Source: CAD feature listing. Evaluate the final solid. Frame: model axes, mm. Face numbers are marked on the shaded views. Coordinates: 2 decimals unless noted, no trailing zeros. Order: outer loops, then holes, each group sorted by start corner. A loop starts at its lowest first (then second) coordinate and runs counter-clockwise, first axis right, second up. Notation, with made-up numbers: (-4, 27) -> (41, 27) arc R25 ccw to (41, 47) -> close; hole circle Ø1 at (-17, -3.75). An arc over 180 degrees is marked (long way). Put each result on its own line as item: value.
from build123d import *

# Parameters (mm, degrees)
F1_DEPTH       = 3.175
F3_DEPTH       = 2.667
F4_SIZE        = 0.127
F5_D           = 1.524
F5_CSINK_D     = 4.826
F5_CSINK_ANGLE = 90
F6_W           = 1.058334
F6_H           = 6.35
F7_DEPTH       = 0.762


with BuildPart() as f1:
    # F0 (on Front) → F1 (new body)
    with BuildSketch(Plane.XZ):
        Polygon((4.758054, 5.239753), (-4.758054, 5.239753), (-4.758054, -15.383445), (-4.250054, -15.383445), (-1.773554, -15.383445), (-1.773554, -14.527198), (1.773554, -14.527198), (1.773554, -15.383445), (4.201267, -15.383445), (4.758054, -15.383445), align=None)
    extrude(amount=F1_DEPTH)

    # F0 (on Front) → F3 (join)
    with BuildSketch(Plane.XZ):
        Polygon((-1.773554, -15.383445), (-4.250054, -15.383445), (-4.250054, -19.304393), (-3.246823, -20.32), (3.185267, -20.32), (4.201267, -19.304393), (4.201267, -15.383445), (1.773554, -15.383445), (1.773554, -14.527198), (-1.773554, -14.527198), align=None)
    extrude(amount=F3_DEPTH)

    # F4
    f4_edges = [f1.edges().sort_by_distance(p)[0] for p in [
        (0, -3.175, 5.239753),
        (-4.758054, -3.175, -5.071846),
        (-4.758054, -1.5875, 5.239753),
        (-4.758054, 0, -5.071846),
        (4.758054, -3.175, -5.071846),
        (4.758054, 0, -5.071846),
        (4.758054, -1.5875, 5.239753),
        (0, 0, 5.239753),
        (-4.250054, -2.667, -17.343919),
        (4.201267, -2.667, -17.343919),
        (4.201267, 0, -17.343919),
        (-4.250054, 0, -17.343919),
        (3.693267, -2.667, -19.812197),
        (-0.030778, -2.667, -20.32),
        (-3.748439, -2.667, -19.812197),
        (-3.748439, 0, -19.812197),
        (-0.030778, 0, -20.32),
        (3.693267, 0, -19.812197),
    ]]
    chamfer(f4_edges, length=F4_SIZE)

    # F5 (through all)
    with Locations(Plane.XZ.offset(3.175)):
        with Locations((0, 0)):
            CounterSinkHole(F5_D / 2, F5_CSINK_D / 2, counter_sink_angle=F5_CSINK_ANGLE)

    # F6 (on face) → F7 (cut)
    with BuildSketch(Plane.XZ.offset(3.175)):
        with Locations((0, -7.352567)):
            Rectangle(F6_W, F6_H)
    extrude(amount=-F7_DEPTH, mode=Mode.SUBTRACT)


solid = f1.part
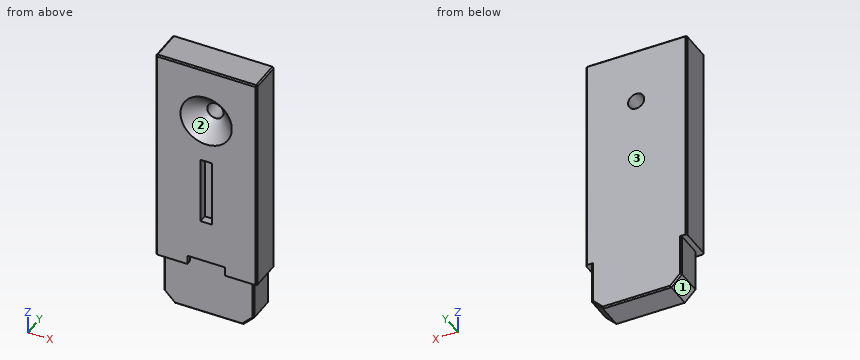
1. Ray query, line 1 along Z through (x, y) = (0, -0.3); line 2 along X through (y, z) = (-0.7, 0); line 3 along Z through (x, y) = (-3, -2.85). Return the intervals inside material, ascending.
Numbers:
line 1: z = -20.32 to -0.76, 0.76 to 5.24
line 2: x = -4.76 to -0.76, 0.76 to 4.76
line 3: z = -15.38 to 5.24
2. Cut plane D-D on y = -2. Output: boundary loops of the cut face in (x, z), plus the area to 3 significant figures.
Numbers:
outline: (-4.76, -15.38) -> (-4.25, -15.38) -> (-4.25, -19.3) -> (-3.25, -20.32) -> (3.19, -20.32) -> (4.2, -19.3) -> (4.2, -15.38) -> (4.76, -15.38) -> (4.76, 5.11) -> (4.63, 5.24) -> (-4.63, 5.24) -> (-4.76, 5.11) -> close; hole circle Ø2.48 at (0, 0)
area: 232 mm2
3. Cut plane A-A on z = 0. Output: boundary loops of the cut face in (x, y) (3 decimals), plus the area to 3 significant figures.
Numbers:
outline: (-4.758, -3.048) -> (-4.631, -3.175) -> (-2.413, -3.175) -> (-0.762, -1.524) -> (-0.762, 0) -> (-4.631, 0) -> (-4.758, -0.127) -> close; (0.762, -1.524) -> (2.413, -3.175) -> (4.631, -3.175) -> (4.758, -3.048) -> (4.758, -0.127) -> (4.631, 0) -> (0.762, 0) -> close
area: 22.6 mm2
4. Cut plane B-B on x = 0. Output: boundary loops of the cut face in (y, z) (3 decimals).
Numbers:
outline: (-3.175, -14.527) -> (-2.667, -14.527) -> (-2.667, -20.193) -> (-2.54, -20.32) -> (-0.127, -20.32) -> (0, -20.193) -> (0, -0.762) -> (-1.524, -0.762) -> (-3.175, -2.413) -> (-3.175, -4.178) -> (-2.413, -4.178) -> (-2.413, -10.528) -> (-3.175, -10.528) -> close; (-3.175, 2.413) -> (-1.524, 0.762) -> (0, 0.762) -> (0, 5.113) -> (-0.127, 5.24) -> (-3.048, 5.24) -> (-3.175, 5.113) -> close
5. First-contact query: pin 1 (0.6 mm diameter, centred on x = -0.5, y = -3, fed in from -Z); pin 2 (3 mm diameter, centred on x = 0.5, z = -18, fed in from -Y); pin 3 (1.9 mm diameter, centred on y = -1, z = -17, fed in from -X). Flat tips, straight axial feed; report the tip coordinate or a pass-through.
Numbers:
pin 1: stops at z = -14.53
pin 2: stops at y = -2.67
pin 3: stops at x = -4.25
6. Cut plane C-C on z = -7.5. Output: boundary loops of the cut face in (x, y) (3 decimals).
Numbers:
outline: (-4.758, -3.048) -> (-4.631, -3.175) -> (-0.529, -3.175) -> (-0.529, -2.413) -> (0.529, -2.413) -> (0.529, -3.175) -> (4.631, -3.175) -> (4.758, -3.048) -> (4.758, -0.127) -> (4.631, 0) -> (-4.631, 0) -> (-4.758, -0.127) -> close
7. Pull-direction query (X, two-part tool) for the marked faces 1, 2 and 3; classes: pulls with the +X half, pulls with the -X half, needs draft (parallel to the pull), parting line crosses it, or undercut.
Numbers:
face 1: pulls with the -X half
face 2: undercut
face 3: needs draft
